Here's how the part is built. I have some questions about the finished solid (model axes, mm). A direction names the side the tool comes from. Round coordinates to 2 decimals unless told otherwise and drop trailing zeros. Loops run counter-clockwise (first coordinate to the right, second up) from the corner with the lowest first, then second, coordinate; pieces in that order, holes last. Notation, with made-up numbers: M -3,29.5 L 47,29.5 A32 ccw 47,68.5 Z; hole C 16.25,78 d11. An arc over 180 degrees is marked long. Use a Markdown table: item, result.
```python
from build123d import *

# Parameters (mm, degrees)
SKETCH1_W           = 92
SKETCH1_H           = 31
BOSS_EXTRUDE1_DEPTH = 46
SKETCH2_R           = 103
SKETCH2_R_2         = 73
CUT_EXTRUDE1_DEPTH  = 47
SKETCH7_R           = 1.2
CUT_EXTRUDE5_DEPTH  = 47
CUT_EXTRUDE2_DEPTH  = 47
SKETCH5_R           = 42.5
CUT_EXTRUDE4_DEPTH  = 17.103780853
CUT_EXTRUDE6_START  = -2
CUT_EXTRUDE6_DEPTH  = 2.2
SKETCH9_W           = 5
SKETCH9_H           = 3.4
CUT_EXTRUDE7_DEPTH  = 17.103780953
CUT_EXTRUDE7_TAPER  = -4


with BuildPart() as part:
    # Sketch1 → Boss-Extrude1 (new body)
    with BuildSketch(Plane(origin=(0, 0, 0), x_dir=(1, 0, 0), z_dir=(0, 1, 0))):
        Rectangle(SKETCH1_W, SKETCH1_H)
    extrude(amount=BOSS_EXTRUDE1_DEPTH)

    # Sketch2 → Cut-Extrude1 (cut, through all)
    with BuildSketch(Plane(origin=(0, 46, 0), x_dir=(1, 0, 0), z_dir=(0, 1, 0))):
        with Locations((0, -53.5)):
            Circle(SKETCH2_R)
        with Locations((0, -53.5)):
            Circle(SKETCH2_R_2, mode=Mode.SUBTRACT)
    extrude(amount=-CUT_EXTRUDE1_DEPTH, mode=Mode.SUBTRACT)

    # Sketch7 → Cut-Extrude5 (cut, through all)
    with BuildSketch(Plane.XZ):
        with Locations((-32, -7.5)):
            Circle(SKETCH7_R)
        with Locations((32, -7.5)):
            Circle(SKETCH7_R)
    extrude(amount=-CUT_EXTRUDE5_DEPTH, mode=Mode.SUBTRACT)

    # Sketch3 → Cut-Extrude2 (cut, through all)
    with BuildSketch(Plane(origin=(0, 46, 0), x_dir=(1, 0, 0), z_dir=(0, 1, 0))):
        with BuildLine():
            Line((-37.855118544, 5.5), (37.855118544, 5.5))
            ThreePointArc((37.855118544, 5.5), (0, -123.6), (-37.855118544, 5.5))
        make_face()
    extrude(amount=-CUT_EXTRUDE2_DEPTH, mode=Mode.SUBTRACT)

    # Sketch5 → Cut-Extrude4 (cut, through all)
    with BuildSketch(Plane(origin=(0, 0, -15.5), x_dir=(-1, 0, 0), z_dir=(0, 0, -1))):
        with Locations((0, 46)):
            Circle(SKETCH5_R)
    extrude(amount=-CUT_EXTRUDE4_DEPTH, mode=Mode.SUBTRACT)

    # Sketch8 → Cut-Extrude6 (cut)
    with BuildSketch(Plane.XZ.offset(CUT_EXTRUDE6_START)):
        Polygon((-34.523561667, -7.229062977), (-33.183568052, -9.55), (-30.816431948, -9.55), (-29.904759513, -7.970937023), (-29.904759513, -4.97225781), (-34.523561667, -4.97225781), align=None)
        Polygon((29.904759513, -4.97225781), (29.904759513, -7.970937023), (30.816431948, -9.55), (33.183568052, -9.55), (34.523561667, -7.229062977), (34.523561667, -4.97225781), align=None)
    extrude(amount=-CUT_EXTRUDE6_DEPTH, mode=Mode.SUBTRACT)

    # Sketch9 → Cut-Extrude7 (cut, through all)
    with BuildSketch(Plane(origin=(0, 0, -15.5), x_dir=(-1, 0, 0), z_dir=(0, 0, -1))):
        with Locations((-14.732750576, 1.7)):
            Rectangle(SKETCH9_W, SKETCH9_H)
    extrude(amount=-CUT_EXTRUDE7_DEPTH, taper=CUT_EXTRUDE7_TAPER, mode=Mode.SUBTRACT)


solid = part.part
```
Q1. Will these pins go through, and if not, where does the flat tip stop? P1, Ø0.7, axis at x = -32.5, y = 3.5, coming from the +Z side; P2, Ø2, axis at y = 26.5, z = -5, coming from the +X side (3 decimals); P3, Ø1.4, axis at x = 32, z = -7.5, coming from the -Y side; P4, Ø0.5, axis at y = 3.5, z = -6.5, coming from the -X side.
Return value:
| item | result |
|---|---|
| P1 | stops at z = -9.55 |
| P2 | stops at x = 44.975 |
| P3 | passes through |
| P4 | stops at x = -41.94 |
Q2. Imagine slicing it at A-A, the plane y = 8.5. Please give me the cut outline in (x, z), then the cut area to 3 significant figures.
Return value:
| item | result |
|---|---|
| outline | M -46,-3.18 A73 ccw -23.83,-15.5 L -20,-15.5 L -20,-5.5 L -37.86,-5.5 A70.1 cw -46,0.6 Z; M 20,-15.5 L 23.83,-15.5 A73 ccw 46,-3.18 L 46,0.6 A70.1 cw 37.86,-5.5 L 20,-5.5 Z; hole C -32,-7.5 d2.4; hole C 32,-7.5 d2.4 |
| area | 323 mm^2 |
Q3. We'd pull the mould along Y, two halves only. Please class faces 1 (the flat face through (28, 0, -9)), 2 (the flat face through (-30.367, 3.085, -8.772)), 3 (the cylindrical face through (-30.855, 0.986, -7.14)): pulls with the +Y half, pulls with the -Y half, needs draft (parallel to the pull), parting line crosses it, or undercut.
Return value:
| item | result |
|---|---|
| face 1 | pulls with the -Y half |
| face 2 | undercut |
| face 3 | needs draft |
Q4. Imagine slicing it at D-D, the plane y = 15.5. Please give me the cut outline in (x, z).
Return value:
| item | result |
|---|---|
| outline | M -46,-3.18 A73 ccw -29.6,-13.23 L -29.6,-5.5 L -37.86,-5.5 A70.1 cw -46,0.6 Z; M 29.6,-13.23 A73 ccw 46,-3.18 L 46,0.6 A70.1 cw 37.86,-5.5 L 29.6,-5.5 Z; hole C -32,-7.5 d2.4; hole C 32,-7.5 d2.4 |
Q5. Imagine slicing it at C-C, the plane y = 38. Please give me the cut outline in (x, z), then the cut area to 3 significant figures.
Return value:
| item | result |
|---|---|
| outline | M -46,-3.18 A73 ccw -41.74,-6.39 L -41.74,-2.82 A70.1 cw -46,0.6 Z; M 41.74,-6.39 A73 ccw 46,-3.18 L 46,0.6 A70.1 cw 41.74,-2.82 Z |
| area | 31.3 mm^2 |
Q6. I need wall thicknesses on line 1 (Z direction, x = 22, y = 8); line 2 (X direction, y = 7.5, z = -3); line 3 (X direction, y = 16, z = -8.5). Which ranges of each line are inside material? Lowest first, please. Write a range as from..to.
Return value:
| item | result |
|---|---|
| line 1 | z = -15.5..-5.5 |
| line 2 | x = -46..-41.49, 41.49..46 |
| line 3 | x = -38.54..-32.66, -31.34..-30.1, 30.1..31.34, 32.66..38.54 |
Q7. Imagine slicing it at B-B, the plane x = 32. Please give me the cut outline in (y, z).
Return value:
| item | result |
|---|---|
| outline | M 0,-12.11 L 18.03,-12.11 L 18.03,-8.7 L 4.2,-8.7 L 4.2,-9.55 L 2,-9.55 L 2,-8.7 L 0,-8.7 Z; M 0,-6.3 L 2,-6.3 L 2,-5.5 L 0,-5.5 Z; M 4.2,-6.3 L 18.03,-6.3 L 18.03,-5.5 L 4.2,-5.5 Z |
Q8. For faces 4 (the flat face through (32, 3, -9.55)), 5 (the cylindrical face through (-42.1, 18.21, -2.55)), 6 (the cylindrical face through (0.93, 3.51, -8.97)), which set-ups out of +Z, -Z, +X, -X, +Y, -Y let a thin tool reach every point of the face, with its end or its side?
Return value:
| item | result |
|---|---|
| face 4 | +Z |
| face 5 | +Z, +Y, -Y |
| face 6 | +Z, -Z, +Y |
